Autodesk Inventor part; units mm, degrees
ref_plane "YZ Plane" through (0, 0, 0) normal (1, 0, 0) x (0, 1, 0)
ref_plane "XZ Plane" through (0, 0, 0) normal (0, 1, 0) x (-1, 0, 0)
ref_plane "XY Plane" through (0, 0, 0) normal (0, 0, 1) x (1, 0, 0)
sketch "Sketch1" plane through (0, 0, 0) normal (0, 1, 0) x (-1, 0, 0)
  circle A0 centre (-14.3247, -0.0006) radius 2.1844
  circle A1 centre (-1.6247, -0.0006) radius 2.1844
  circle A2 centre (3.6787, 11.5391) radius 2.1844
  circle A3 centre (3.6787, 11.5391) radius 6.35
  circle A4 centre (-1.6247, -0.0006) radius 6.35
  circle A5 centre (-14.3247, -0.0006) radius 6.35
  line L0 (-1.6247, -6.3506) -> (-14.3247, -6.3506)
  line L1 (4.1452, -2.6523) -> (9.4485, 8.8874)
  line L2 (-2.0912, 14.1907) -> (-7.3945, 2.651)
  line L3 (-1.6247, 6.3494) -> (-14.3247, 6.3494)
  point P0 (0, 0)
  point P1 (0.252, 16.8851)
  point P2 (-17.7513, 5.3454)
  point P3 (-7.9747, -0.0006)
  point P4 (1.027, 5.7692)
  point P5 (-5.6949, 6.3494)
  dimension "d0" = 12.7
  dimension "d1" = 12.7
  dimension "d2" = 12.7
extrude "Extrusion1" add sketch "Sketch1" along normal blind 1.5875
properties part number "lbL-channelSupport"
Geometry: final body of the model. Coordinates: model frame, mm. Coordinates: 2 decimals unless noted, no trailing zeros. Order: outer loops, then holes, each group sorted by start corner. A loop starts at its lowest first (then second) coordinate and runs counter-clockwise, first axis right, second up.
1) Ray query, probe 1 along Z at (x, y) = (0.5, 0.6); probe 2 along X at (y, z) = (0.65, 0.5); probe 3 along Z at (x, y) = (0, 0.8). Return the intervals inside material, ascending.
Result sheet:
probe 1: z = -6.25 to -1.87, 1.87 to 16.32
probe 2: x = -5.59 to -0.5, 3.75 to 12.2, 16.45 to 20.65
probe 3: z = -6.14 to -1.46, 1.46 to 16.71
2) Section D-D (x = 9). Return loops of the section in (y, z), then the cut area to 3 significant figures.
Result sheet:
outline: (0, -6.35) - (1.59, -6.35) - (1.59, 6.35) - (0, 6.35) - close
area: 20.2 mm2
3) Section C-C (y = 1.1). Return loops of the section in (x, z), then the cut area to 3 significant figures.
Result sheet:
outline: (-9.45, 8.89) - (-4.15, -2.65) arc R6.35 ccw to (1.62, -6.35) - (14.32, -6.35) arc R6.35 ccw to (14.32, 6.35) - (5.69, 6.35) - (2.09, 14.19) arc R6.35 ccw to start; hole circle Ø4.37 at (-3.68, 11.54); hole circle Ø4.37 at (1.62, 0); hole circle Ø4.37 at (14.32, 0)
area: 401 mm2
4) Draft query along X for faces 1 (the cylindrical face through (-6.203, 0.783, 17.366)), 2 (the cylindrical face through (-3.205, 0.783, 13.672)), 3 (the flat face through (10, 1, 6.349)), 4 (the cylindrical face through (12.31, 0.78, 0.84)). Return one class per face: released by +X, released by -X, zero draft, split by the parting line, or undercut.
Result sheet:
face 1: split by the parting line
face 2: undercut
face 3: zero draft
face 4: undercut
5) Section A-A (x = 16). Return loops of the section in (y, z).
Result sheet:
outline: (0, -6.13) - (1.59, -6.13) - (1.59, -1.4) - (0, -1.4) - close; (0, 1.4) - (1.59, 1.4) - (1.59, 6.12) - (0, 6.12) - close
6) First-contact query: P1, Ø7, axis at x = -3.68, z = 11.54, coming from the -Y side; P2, Ø0.8, axis at x = 12, y = 1, coming from the +Z side. Flat tips, straight axial feed; report the tip coordinate or a pass-through.
Result sheet:
P1: stops at y = 0
P2: stops at z = 6.35
7) Section B-B (z = 12.25). Return loops of the section in (x, y), then the cut area to 3 significant figures.
Result sheet:
outline: (-9.99, 0) - (-5.74, 0) - (-5.74, 1.59) - (-9.99, 1.59) - close; (-1.61, 0) - (2.98, 0) - (2.98, 1.59) - (-1.61, 1.59) - close
area: 14.0 mm2
